```python
from build123d import *

# Parameters (mm, degrees)
SKETCH_1_W          = 50
SKETCH_1_H          = 27
EXTRUDE_1_DEPTH     = 35
SKETCH_2_W          = 50
SKETCH_2_H          = 21
CUT_EXTRUDE_1_DEPTH = 15
SKETCH_3_R          = 1.6
CUT_EXTRUDE_2_DEPTH = 28
SKETCH_4_W          = 14
SKETCH_4_H          = 21
CUT_EXTRUDE_3_DEPTH = 51
EXTRUDE_2_DEPTH     = 50
CUT_EXTRUDE_4_DEPTH = 51
SKETCH_8_R          = 1.6
CUT_EXTRUDE_5_DEPTH = 50


with BuildPart() as part:
    # 草图1 → 凸台-拉伸1 (new body)
    with BuildSketch(Plane.XY):
        with Locations((3.800856531, -0.170235546)):
            Rectangle(SKETCH_1_W, SKETCH_1_H)
    extrude(amount=EXTRUDE_1_DEPTH)

    # 草图2 → 切除-拉伸1 (cut)
    with BuildSketch(Plane.XY.offset(35)):
        with Locations((3.800856531, -0.170235546)):
            Rectangle(SKETCH_2_W, SKETCH_2_H)
    extrude(amount=-CUT_EXTRUDE_1_DEPTH, mode=Mode.SUBTRACT)

    # 草图3 → 切除-拉伸2 (cut, through all)
    with BuildSketch(Plane.XZ.offset(13.670235546)):
        with Locations((-3.699143469, 30)):
            Circle(SKETCH_3_R)
        with Locations((11.300856531, 30)):
            Circle(SKETCH_3_R)
    extrude(amount=-CUT_EXTRUDE_2_DEPTH, mode=Mode.SUBTRACT)

    # 草图4 → 切除-拉伸3 (cut, through all)
    with BuildSketch(Plane.ZY.offset(21.199143469)):
        with Locations((10, -0.170235546)):
            Rectangle(SKETCH_4_W, SKETCH_4_H)
    extrude(amount=-CUT_EXTRUDE_3_DEPTH, mode=Mode.SUBTRACT)

    # 草图6 → 凸台-拉伸2 (add)
    with BuildSketch(Plane(origin=(28.800856531, 0, 0), x_dir=(0, 0, -1), z_dir=(1, 0, 0))):
        Polygon((0, -13.670235546), (50.983856303, -74.430429459), (64.278760969, -63.274679858), (0, 13.329764454), align=None)
    extrude(amount=-EXTRUDE_2_DEPTH)

    # 草图7 → 切除-拉伸4 (cut, through all)
    with BuildSketch(Plane(origin=(28.800856531, 0, 0), x_dir=(0, 0, -1), z_dir=(1, 0, 0))):
        Polygon((60.05226481, -62.904909358), (3, 5.087332196), (3, -12.578324843), (51.353626803, -70.203933301), align=None)
    extrude(amount=-CUT_EXTRUDE_4_DEPTH, mode=Mode.SUBTRACT)

    # 草图8 → 切除-拉伸5 (cut)
    with BuildSketch(Plane(origin=(0, -68.782217432, -57.715133279), x_dir=(-1, 0, 0), z_dir=(0, -0.766044443, -0.64278761))):
        with Locations((-13.800856531, -0.1094253)):
            Circle(SKETCH_8_R)
        with Locations((6.199143469, -0.1094253)):
            Circle(SKETCH_8_R)
    extrude(amount=-CUT_EXTRUDE_5_DEPTH, mode=Mode.SUBTRACT)


solid = part.part
```
Part model, mm, in its own coordinate system. A direction names the side the tool comes from. Coordinates: 2 decimals unless noted, no trailing zeros. Order: outer loops, then holes, each group sorted by start corner. A loop starts at its lowest first (then second) coordinate and runs counter-clockwise, first axis right, second up. Notation, with made-up numbers: (18, 26.25) - (77, 26.25) arc R18 cw to (77, 42.25) - close; hole circle Ø9 at (66, 80.5). An arc over 180 degrees is marked (long way). Return JSON: item names as keys, results as strings. Group by question number.
Item 1: Cut at B-B (x = -11). List the corners of the cut face in (y, z).
Item 2: Cut at D-D (y = -4.5). List the corners of the cut face in (x, z), plus the area to 3 significant figures.
Item 3: Pull direction Y, two halves, no side cores. Call faces 1 (the face through (4.151, -29.385, -31.925)), 2 (the face through (4.15, -43.63, -25.14)), 3 (the face through (-21.199, -24, -11)): pulls with the +Y half, pulls with the -Y half, needs draft (parallel to the pull), parting line crosses it, or undercut.
Item 4: Drill centre lines: probe 1 along Y at (x, z) = (18.5, 14.5); probe 2 along Y at (x, z) = (-14.5, 0.5); probe 3 along Z at (x, y) = (25, 8). Where is each one in solid material? Low to high. Write a range as from..to.
Item 5: Cut at A-A (z = 10). List the corners of the cut face in (x, y), plus the area to 3 significant figures.
Item 6: Cut at C-C (z = 30). List the corners of the cut face in (x, y), plus the area to 3 significant figures.
Item 7: Pin check, flat tips, straight feed: pin 1 (3 mm diameter, centred on x = 7.5, z = -10, fed in from +Y); pin 2 (23 mm diameter, centred on x = 10, y = -1.5, fed in from -Z); pin 3 (6 mm diameter, centred on x = 11, z = -42.5, fed in from -Y) (3 decimals). Stop position of each tip, or through.
Item 8: Which spindle directions (+Z, -Z, +X, -X, +Y, -Y) get a long thin tool onto all of the face, cutting with end or side? Do faces 4 (the face through (3, -10.67, 10)), 5 (the face through (3, -13.67, 17)), 6 (the face through (3, 13.33, 17)), 7 (the face through (3, 10.33, 28)), 8 (the face through (-3.907, 11.809, 31.586)). Say none if no direction does.
Check values:
{
 "1": {"outline": "(-74.43, -50.98) - (-63.27, -64.28) - (13.33, 0) - (13.33, 35) - (10.33, 35) - (10.33, 20) - (-10.67, 20) - (-10.67, 35) - (-13.67, 35) - (-13.67, 0) - close; hole (-70.2, -51.35) - (-62.9, -60.05) - (5.09, -3) - (-12.58, -3) - close; hole (-10.67, 3) - (10.33, 3) - (10.33, 17) - (-10.67, 17) - close"},
 "2": {"outline": "(-21.2, -14.96) - (28.8, -14.96) - (28.8, -11.04) - (-21.2, -11.04) - close; (-21.2, -3) - (28.8, -3) - (28.8, 3) - (-21.2, 3) - close; (-21.2, 17) - (28.8, 17) - (28.8, 20) - (-21.2, 20) - close", "area": "646 mm2"},
 "3": {"face 1": "undercut", "face 2": "pulls with the -Y half", "face 3": "needs draft"},
 "4": {"probe 1": "y = -13.67..-10.67, 10.33..13.33", "probe 2": "y = -13.67..13.33", "probe 3": "z = -4.47..3, 17..20"},
 "5": {"outline": "(-21.2, -13.67) - (28.8, -13.67) - (28.8, -10.67) - (-21.2, -10.67) - close; (-21.2, 10.33) - (28.8, 10.33) - (28.8, 13.33) - (-21.2, 13.33) - close", "area": "300 mm2"},
 "6": {"outline": "(-21.2, -13.67) - (-5.3, -13.67) - (-5.3, -10.67) - (-21.2, -10.67) - close; (-21.2, 10.33) - (-5.3, 10.33) - (-5.3, 13.33) - (-21.2, 13.33) - close; (-2.1, -13.67) - (9.7, -13.67) - (9.7, -10.67) - (-2.1, -10.67) - close; (-2.1, 10.33) - (9.7, 10.33) - (9.7, 13.33) - (-2.1, 13.33) - close; (12.9, -13.67) - (28.8, -13.67) - (28.8, -10.67) - (12.9, -10.67) - close; (12.9, 10.33) - (28.8, 10.33) - (28.8, 13.33) - (12.9, 13.33) - close", "area": "262 mm2"},
 "7": {"pin 1": "stops at y = 3.2", "pin 2": "stops at z = -22.09", "pin 3": "stops at y = -67.895"},
 "8": {"face 4": "+X, -X", "face 5": "+Z, +X, -X, -Y", "face 6": "+Z, -Z, +X, -X, +Y", "face 7": "+Z, +X, -X", "face 8": "+Y, -Y"}
}
